Check sheet for the modelled part. Datum: model origin and axes. Units: mm. A direction names the side the tool comes from. Give positions to 0.01 mm unless a question says otherwise; leave off trailing zeros. Write each loop counter-clockwise with the first axis right and the second up, starting at its lowest first coordinate (ties: lowest second). Pieces come first, ordered by that corner, then holes.
from build123d import *

# Parameters (mm, degrees)
SALIENTE_EXTRUIR1_DEPTH = 5.25
CORTAR_EXTRUIR1_DEPTH   = 1
CORTAR_EXTRUIR2_DEPTH   = 0.5
REDONDEO1_R             = 0.25
CROQUIS4_W              = 0.5
CROQUIS4_H              = 0.5
SALIENTE_EXTRUIR2_DEPTH = 8
CROQUIS5_R              = 1
CORTAR_EXTRUIR3_DEPTH   = 0.5
C_PULA1_FACE_RADIUS     = 1
C_PULA1_HEIGHT          = 1


# Read off the part's stored shape, not the designer's step: Cúpula2
with BuildPart() as part:
    # Croquis2 → Saliente-Extruir1 (new body)
    with BuildSketch(Plane(origin=(0, 0, 0), x_dir=(0, 0, -1), z_dir=(1, 0, 0))):
        Polygon((-3.15, -3.15), (3.15, -3.15), (3.15, -0.65), (2.65, -0.65), (2.65, 0.65), (3.15, 0.65), (3.15, 3.15), (-3.15, 3.15), (-3.15, 0.65), (-2.65, 0.65), (-2.65, -0.65), (-3.15, -0.65), align=None)
    extrude(amount=SALIENTE_EXTRUIR1_DEPTH)

    # Croquis2<4> → Cortar-Extruir1 (cut)
    with BuildSketch(Plane(origin=(0, 0, 0), x_dir=(0, 0, -1), z_dir=(1, 0, 0))):
        Polygon((-2.65, -2.65), (-2.65, -1.15), (-2.15, -1.15), (-2.15, 1.15), (-2.65, 1.15), (-2.65, 2.65), (2.65, 2.65), (2.65, 1.15), (2.15, 1.15), (2.15, -1.15), (2.65, -1.15), (2.65, -2.65), align=None)
    extrude(amount=CORTAR_EXTRUIR1_DEPTH, mode=Mode.SUBTRACT)

    # Croquis3 → Cortar-Extruir2 (cut)
    with BuildSketch(Plane(origin=(5.25, 0, 0), x_dir=(0, 0, -1), z_dir=(1, 0, 0))):
        Polygon((2.65, 1.15), (2.65, 2.65), (-2.65, 2.65), (-2.65, 1.15), (-2.15, 1.15), (-2.15, -1.15), (-2.65, -1.15), (-2.65, -2.65), (2.65, -2.65), (2.65, -1.15), (2.15, -1.15), (2.15, 1.15), align=None)
    extrude(amount=-CORTAR_EXTRUIR2_DEPTH, mode=Mode.SUBTRACT)

    # Redondeo1
    redondeo1_edges = [part.edges().sort_by_distance(p)[0] for p in [
        (4.75, 1.9, -2.65),
        (4.75, 1.15, -2.4),
        (4.75, 0, -2.15),
        (4.75, -1.15, -2.4),
        (4.75, -1.9, -2.65),
        (4.75, -2.65, 0),
        (4.75, -1.9, 2.65),
        (4.75, -1.15, 2.4),
        (4.75, 0, 2.15),
        (4.75, 1.15, 2.4),
        (4.75, 1.9, 2.65),
        (4.75, 2.65, 0),
    ]]
    fillet(redondeo1_edges, radius=REDONDEO1_R)

    # Croquis4 → Saliente-Extruir2 (add)
    with BuildSketch(Plane(origin=(4.75, 0, 0), x_dir=(0, 0, -1), z_dir=(1, 0, 0))):
        with Locations((-1.256816684, 1.4)):
            Rectangle(CROQUIS4_W, CROQUIS4_H)
        with Locations((1.243183316, 1.4)):
            Rectangle(CROQUIS4_W, CROQUIS4_H)
        with Locations((1.243183316, -1.6)):
            Rectangle(CROQUIS4_W, CROQUIS4_H)
        with Locations((-1.256816684, -1.6)):
            Rectangle(CROQUIS4_W, CROQUIS4_H)
    extrude(amount=SALIENTE_EXTRUIR2_DEPTH)

    # Croquis5 → Cortar-Extruir3 (cut)
    with BuildSketch(Plane.ZY.offset(-1)):
        with Locations((0, 1.5)):
            Circle(CROQUIS5_R)
        with Locations(Location((0, -1.5, 0), (0, 0, 180))):
            Circle(CROQUIS5_R)
    extrude(amount=-CORTAR_EXTRUIR3_DEPTH, mode=Mode.SUBTRACT)

    # Cúpula1: a dome of height H over a round flat face of radius A is a cap of a sphere of radius (A * A + H * H) / (2 * H)
    c_pula1_r = (C_PULA1_FACE_RADIUS * C_PULA1_FACE_RADIUS + C_PULA1_HEIGHT * C_PULA1_HEIGHT) / (2 * C_PULA1_HEIGHT)
    c_pula1_base = Plane((1.5, 1.5, 0), z_dir=(-1, 0, 0))
    with Locations(c_pula1_base.offset(C_PULA1_HEIGHT - c_pula1_r)):
        c_pula1_ball = Sphere(c_pula1_r, mode=Mode.PRIVATE)
    add(split(c_pula1_ball, bisect_by=c_pula1_base, keep=Keep.TOP, mode=Mode.PRIVATE))

    # Cúpula2 outline → Cúpula2 (revolve)
    with BuildSketch(Plane(origin=(0, -1.5, 0), x_dir=(0, 1, 0), z_dir=(0, 0, -1))):
        with BuildLine():
            Line((0, 1.500000001), (0, 0.5))
            ThreePointArc((0, 0.5), (0.707106782, 0.792893219), (1, 1.500000001))
            Line((1, 1.500000001), (0, 1.500000001))
        make_face()
    revolve(axis=Axis((0, -1.5, 0), (1, 0, 0)))


solid = part.part
1) Sectioned sample at A-A on x = 6. Record the boundary of the cut face in (y, z).
2) Scan lines: L1, parallel to Y at x = 3.5, z = 2.75; L2, parallel to X at y = 2.5, z = 2.75; L3, parallel to X at y = 1, z = -1. Record each from-to range of solid material in increasing order.
3) Sectioned sample at C-C on y = 0. Record the boundary of the cut face in (x, z), then the cut area to 3 significant figures.
4) Sectioned sample at B-B on z = -1.25. Record the boundary of the cut face in (x, y), then the cut area to 3 significant figures.
5) Access from +Z, -Z, +X, -X, +Y, -Y to the whole of each face (thin tool, end or side, straight path). Record for faces 1 (the flat face through (3, 0, -2.65)), 2 (the flat face through (3, 2, 3.15)), 3 (the flat face through (0.5, 1.9, -2.65)), 4 (the flat face through (3, -2, -3.15)), 5 (the flat face through (3, 0, 2.65)).
6) Gauge pin test, flat ends, axial feed: pin 1 (2 mm diameter, centred on x = 10, y = -0.5, fed in from -Z); pin 2 (2.5 mm diameter, centred on y = 0, z = 0, fed in from -X). Record the tip position at first contact, or that the pin passes through.
7) Sectioned sample at D-D on x = 4.25. Record the boundary of the cut face in (y, z), then the cut area to 3 significant figures.
Answers below:
1. outline: (-1.85, -1.49) - (-1.35, -1.49) - (-1.35, -0.99) - (-1.85, -0.99) - close; (-1.85, 1.01) - (-1.35, 1.01) - (-1.35, 1.51) - (-1.85, 1.51) - close; (1.15, -1.49) - (1.65, -1.49) - (1.65, -0.99) - (1.15, -0.99) - close; (1.15, 1.01) - (1.65, 1.01) - (1.65, 1.51) - (1.15, 1.51) - close
2. L1: y = -3.15 to -0.65, 0.65 to 3.15
2. L2: x = 0 to 5.25
2. L3: x = 1 to 4.75
3. outline: (0, -2.65) - (5.25, -2.65) - (5.25, -2.15) - (5, -2.15) arc R0.25 cw to (4.75, -1.9) - (4.75, 1.9) arc R0.25 cw to (5, 2.15) - (5.25, 2.15) - (5.25, 2.65) - (0, 2.65) - (0, 2.15) - (1, 2.15) - (1, -2.15) - (0, -2.15) - close
3. area: 21.4 mm2
4. outline: (0, -3.15) - (5.25, -3.15) - (5.25, -2.65) - (5, -2.65) arc R0.25 cw to (4.75, -2.4) - (4.75, -1.85) - (12.75, -1.85) - (12.75, -1.35) - (4.75, -1.35) - (4.75, 1.15) - (12.75, 1.15) - (12.75, 1.65) - (4.75, 1.65) - (4.75, 2.4) arc R0.25 cw to (5, 2.65) - (5.25, 2.65) - (5.25, 3.15) - (0, 3.15) - (0, 2.65) - (1, 2.65) - (1, -2.65) - (0, -2.65) - close
4. area: 33.2 mm2
5. face 1: -Z, +X, -X
5. face 2: +Z, +X, -X, +Y, -Y
5. face 3: -X
5. face 4: -Z, +X, -X, +Y, -Y
5. face 5: +Z, +X, -X
6. pin 1: stops at z = -1.49
6. pin 2: stops at x = 0.53
7. outline: (-3.15, -3.15) - (-0.65, -3.15) - (-0.65, -2.65) - (0.65, -2.65) - (0.65, -3.15) - (3.15, -3.15) - (3.15, 3.15) - (0.65, 3.15) - (0.65, 2.65) - (-0.65, 2.65) - (-0.65, 3.15) - (-3.15, 3.15) - close
7. area: 38.4 mm2
